from build123d import *

# Parameters (mm, degrees)
SALIENTE_EXTRUIR1_DEPTH   = 150
CROQUIS2_OUTSIDE_W        = 38.098
CROQUIS2_OUTSIDE_H        = 37.48
CROQUIS2_OUTSIDE_R        = 1.8
CORTAR_EXTRUIR2_DEPTH     = 2
CORTAR_EXTRUIR2_DRAFT     = -20
SIMETR_A1_COPY_1_SKETCH_W = 38.098
SIMETR_A1_COPY_1_SKETCH_H = 37.48
SIMETR_A1_COPY_1_SKETCH_R = 1.8
SIMETR_A1_COPY_1_DEPTH    = 2
SIMETR_A1_COPY_1_DRAFT    = -20


with BuildPart() as part:
    # Croquis1 → Saliente-Extruir1 (new body)
    with BuildSketch(Plane.XY):
        Polygon((2.309401077, 0), (1.154700538, 2), (-1.154700538, 2), (-2.309401077, 0), (-1.154700538, -2), (1.154700538, -2), align=None)
    extrude(amount=SALIENTE_EXTRUIR1_DEPTH)


with BuildPart() as cortar_extruir2_tool:
    # Croquis2 outside → Cortar-Extruir2 (with draft: the straight prism first)
    with BuildSketch(Plane.XY.offset(150)):
        Rectangle(CROQUIS2_OUTSIDE_W, CROQUIS2_OUTSIDE_H)
        Circle(CROQUIS2_OUTSIDE_R, mode=Mode.SUBTRACT)
    extrude(amount=-CORTAR_EXTRUIR2_DEPTH)
    # Cortar-Extruir2: the draft: its side faces are tilted about the plane it starts from
    cortar_extruir2_sides = [cortar_extruir2_tool.faces().sort_by_distance(p)[0] for p in [
        (0, -18.74, 149),
        (19.049, 0, 149),
        (0, 18.74, 149),
        (-19.049, 0, 149),
        (-1.8, 0, 149),
    ]]
    draft(cortar_extruir2_sides, Plane.XY.offset(150), CORTAR_EXTRUIR2_DRAFT)


with BuildPart() as part_1:
    add(part.part)

    # Cortar-Extruir2: cut by cortar_extruir2_tool
    add(cortar_extruir2_tool.part, mode=Mode.SUBTRACT)


with BuildPart() as simetr_a1_copy_1_tool:
    # Simetría1 copy 1 sketch → Simetría1 copy 1 (with draft: the straight prism first)
    with BuildSketch(Plane(origin=(0, 0, 0), x_dir=(1, 0, 0), z_dir=(0, 0, -1))):
        Rectangle(SIMETR_A1_COPY_1_SKETCH_W, SIMETR_A1_COPY_1_SKETCH_H)
        Circle(SIMETR_A1_COPY_1_SKETCH_R, mode=Mode.SUBTRACT)
    extrude(amount=-SIMETR_A1_COPY_1_DEPTH)
    # Simetría1 copy 1: the draft: its side faces are tilted about the plane it starts from
    simetr_a1_copy_1_sides = [simetr_a1_copy_1_tool.faces().sort_by_distance(p)[0] for p in [
        (0, -18.74, 1),
        (19.049, 0, 1),
        (0, 18.74, 1),
        (-19.049, 0, 1),
        (-1.8, 0, 1),
    ]]
    draft(simetr_a1_copy_1_sides, Plane(origin=(0, 0, 0), x_dir=(1, 0, 0), z_dir=(0, 0, -1)), SIMETR_A1_COPY_1_DRAFT)


with BuildPart() as part_2:
    add(part_1.part)

    # Simetría1 copy 1: cut by simetr_a1_copy_1_tool
    add(simetr_a1_copy_1_tool.part, mode=Mode.SUBTRACT)


solid = part_2.part
Source: CAD feature listing. Evaluate the final solid. Frame: model axes, mm. Coordinates: 2 decimals unless noted, no trailing zeros. Loops run counter-clockwise (first coordinate to the right, second up) from the corner with the lowest first, then second, coordinate; pieces in that order, holes last. Notation, with made-up numbers: (19, 17) - (29, 17) arc R5 cw to (29, 21) - close; hole circle Ø11 at (51, -18). An arc over 180 degrees is marked (long way). Return JSON: item names as keys, results as strings.
Q1. Section A-A, the plane z = 94.5. Return loops of the section in (x, y).
Results:
{"outline": "(-2.31, 0) - (-1.15, -2) - (1.15, -2) - (2.31, 0) - (1.15, 2) - (-1.15, 2) - close"}
Q2. Material intervals for line 1 along Y through (x, z) = (-1.65, 20.5); line 2 along X through (y, z) = (-0.05, 113); line 3 along X through (y, z) = (0.55, 87), sorted ascending.
Results:
{"line 1": "-1.14 to 1.14", "line 2": "-2.28 to 2.28", "line 3": "-1.99 to 1.99"}
Q3. Contact query for flat-ended pins moving along their axis: P1, Ø1, axis at y = 1, z = 70, coming from the -X side; P2, Ø1, axis at x = 0, y = -0.5, coming from the -Z side. Output: stop coordinate, or through.
Results:
{"P1": "x = -2.02", "P2": "z = 0"}
